```python
from build123d import *

# Parameters (mm, degrees)
SKETCH1_R               = 6
BOSS_EXTRUDE1_DEPTH     = 40
CUT_EXTRUDE3_DEPTH      = 1
CUT_EXTRUDE3_DEPTH_BACK = 30


with BuildPart() as part:
    # Sketch1 → Boss-Extrude1 (new body)
    with BuildSketch(Plane(origin=(0, 0, 0), x_dir=(1, 0, 0), z_dir=(0, 1, 0))):
        Circle(SKETCH1_R)
    extrude(amount=BOSS_EXTRUDE1_DEPTH)

    # Sketch2 → Cut-Extrude3 (cut, two sides)
    with BuildSketch(Plane.XZ) as cut_extrude3_sk:
        with BuildLine():
            Line((1.645448267, 2.09), (-1.645448267, 2.09))
            ThreePointArc((-1.645448267, 2.09), (-1.161616892, -2.392957625), (2.66, 0))
            ThreePointArc((2.66, 0), (2.392957625, 1.161616892), (1.645448267, 2.09))
        make_face()
    extrude(amount=CUT_EXTRUDE3_DEPTH, mode=Mode.SUBTRACT)
    extrude(cut_extrude3_sk.sketch, amount=-CUT_EXTRUDE3_DEPTH_BACK, mode=Mode.SUBTRACT)


solid = part.part
```
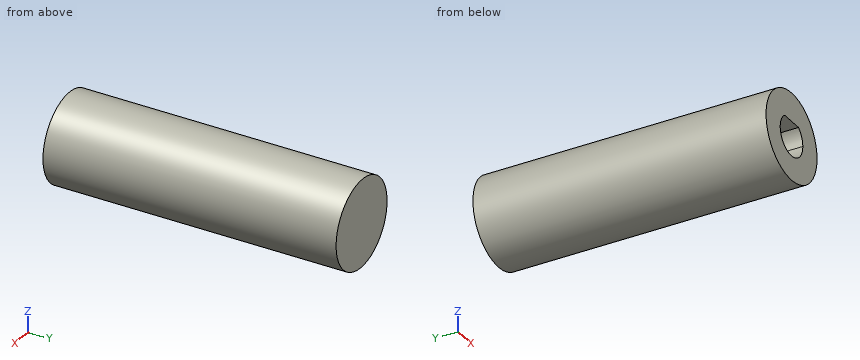
Can you work these out from the model? Positions are in its coordinate system, mm. Give positions to 0.01 mm unless a question says otherwise; leave off trailing zeros. Write each loop counter-clockwise with the first axis right and the second up, starting at its lowest first coordinate (ties: lowest second). Pieces come first, ordered by that corner, then holes. Notation, with made-up numbers: (83, 76.25) -> (112, 76.25) arc R24 cw to (112, 111.25) -> close; hole circle Ø1 at (-28, -28). An arc over 180 degrees is marked (long way). One line per item, written item: value.
Q1. Please list where these lines run through material, in increasing order: line 1 (X direction, y = 20.5, z = 0); line 2 (Z direction, x = 0, y = 19.75); line 3 (Y direction, x = 0.5, z = -1.75). Write a range as [from, to].
Results found:
line 1: x = [-6, -2.66], [2.66, 6]
line 2: z = [-6, -2.66], [2.09, 6]
line 3: y = [30, 40]
Q2. For P1, Ø1, axis at x = -1.5, y = 14.5, coming from the -Z side; P2, Ø1, axis at y = 6, z = -2.5, coming from the +X side; P3, Ø1.4, axis at x = -0.5, z = -1, coming from the -Y side, each with a flat end and sliding along its axis, tell me the tip position at first contact or that it passes through.
Results found:
P1: stops at z = -5.92
P2: stops at x = 5.66
P3: stops at y = 30
Q3. Imagine slicing it at B-B on y = 9. Please give me the cut outline in (x, z).
Results found:
outline: circle Ø12 at (0, 0); hole (-1.65, 2.09) arc R2.66 ccw (long way) to (1.65, 2.09) -> close
Q4. Imagine slicing it at D-D on y = 33.5. Please give me the cut outline in (x, z).
Results found:
outline: circle Ø12 at (0, 0)
Q5. Imagine slicing it at C-C on z = -0.5. Please give me the cut outline in (x, y).
Results found:
outline: (-5.98, 0) -> (-2.61, 0) -> (-2.61, 30) -> (2.61, 30) -> (2.61, 0) -> (5.98, 0) -> (5.98, 40) -> (-5.98, 40) -> close
Q6. Imagine slicing it at A-A on x = 0. Please give me the cut outline in (y, z), and give its area (4 significant figures).
Results found:
outline: (0, -6) -> (40, -6) -> (40, 6) -> (0, 6) -> (0, 2.09) -> (30, 2.09) -> (30, -2.66) -> (0, -2.66) -> close
area: 337.5 mm^2
